from build123d import *

# Parameters (mm, degrees)
SKETCH1_W                   = 240
SKETCH1_H                   = 50
BOSS_EXTRUDE1_DEPTH         = 40
M12X1_75_TAPPED_HOLE1_D     = 10.2
M12X1_75_TAPPED_HOLE1_DEPTH = 20
M12X1_75_TAPPED_HOLE1_TIP   = 3.064389157


with BuildPart() as part:
    # Sketch1 → Boss-Extrude1 (new body)
    with BuildSketch(Plane(origin=(0, 0, 0), x_dir=(1, 0, 0), z_dir=(0, 1, 0))):
        with Locations((120, -25)):
            Rectangle(SKETCH1_W, SKETCH1_H)
    extrude(amount=BOSS_EXTRUDE1_DEPTH)

    # M12x1.75 Tapped Hole1
    with Locations(Plane(origin=(0, 40, 0), x_dir=(1, 0, 0), z_dir=(0, 1, 0))):
        with Locations((20, -25), (220, -25)):
            Hole(M12X1_75_TAPPED_HOLE1_D / 2, depth=M12X1_75_TAPPED_HOLE1_DEPTH)
            with Locations((0, 0, -(M12X1_75_TAPPED_HOLE1_DEPTH + M12X1_75_TAPPED_HOLE1_TIP / 2))):  # 118° drill point
                Cone(0, M12X1_75_TAPPED_HOLE1_D / 2, M12X1_75_TAPPED_HOLE1_TIP, mode=Mode.SUBTRACT)


solid = part.part
Geometry: final body of the model. Coordinates: model frame, mm. A direction names the side the tool comes from. Round coordinates to 2 decimals unless told otherwise and drop trailing zeros. Write each question's results on one line, items separated by ' | '.
Item 1: Material intervals for line 1 along X through (y, z) = (28, 25); line 2 along X through (y, z) = (37.5, 26); line 3 along Z through (x, y) = (20, 32), sorted ascending. Write a range as [from, to].
Completed:
line 1: [0, 14.9], [25.1, 214.9], [225.1, 240] | line 2: [0, 15], [25, 215], [225, 240] | line 3: [0, 19.9], [30.1, 50]
Item 2: Reachability of faces 4 (the flat face through (118, 40, 25)), 5 (the cylindrical face through (215.289, 29.86, 26.953)) from +Z, -Z, +X, -X, +Y, -Y: full face, straight path, thin tool, end or side. Return the list, or none.
Completed:
face 4: +Z, -Z, +X, -X, +Y | face 5: +Y
Item 3: Mould query, pull axis X, two halves, no side actions, for faces 1 (the flat face through (118, 0, 25)), 2 (the cylindrical face through (21, 30, 30)), 3 (the flat face through (240, 20, 25)). Classes: pulls with the +X half, pulls with the -X half, needs draft (parallel to the pull), parting line crosses it, or undercut.
Completed:
face 1: needs draft | face 2: undercut | face 3: pulls with the +X half
Item 4: First-contact query: pin 1 Ø9 at (x, z) = (220, 25) entering from +Y. Flat tip, straight axial feed; report the tip coordinate or a pass-through.
Completed:
pin 1: y = 19.64
